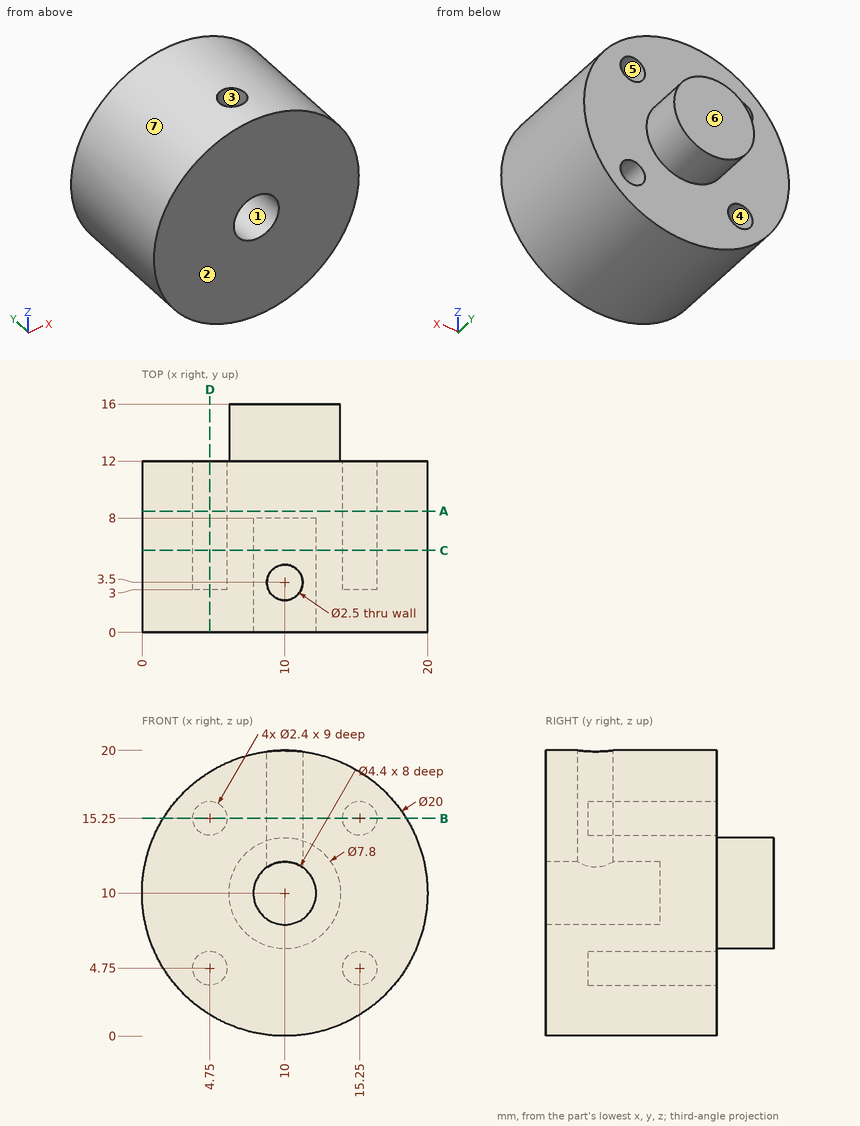
Study the drawing (mm; zero at the part's minimum x, y, z) and answer. A direction names the side the tool comes from. Give positions to 0.01 mm unless a question says otherwise; leave off trailing zeros. Write each loop counter-clockwise with the first axis right and the second up, starting at its lowest first coordinate (ties: lowest second). Pieces come first, ordered by that corner, then holes. Notation, with made-up numbers: (-11.75, 75) -> (19.25, 75) arc R30 ccw to (19.25, 106) -> close; hole circle Ø9 at (38, 75). An arc over 180 degrees is marked (long way). Write item = value, one per line. Start each with the question number.
1) Determine the mould class of the marked faces 5, 6 and 7 for opening direction X: +X half, -X half, draft (parallel to the pull), parting line (faces both ways), or undercut.
2) Each of these flat-tipped pins is pushed along its axis until it touches: pin 1 (5 mm diameter, centred on y = 7.5, z = 14, fed in from -X); pin 2 (1.9 mm diameter, centred on x = 4.75, z = 15.25, fed in from +Y); pin 3 (6 mm diameter, centred on x = 5.5, y = 7.5, fed in from -Z); pin 4 (5.5 mm diameter, centred on x = 10, z = 10, fed in from -Y). Where does it stop, or does it pass through?
3) The part is cut by section D-D, the plane x = 4.75. Determine the outline of the cut face in (y, z).
4) The part is cut by section A-A, the plane y = 8.5. Determine the outline of the cut face in (x, z), and give its area (3 significant figures).
5) The part is cut by section C-C, the plane y = 5.75. Determine the outline of the cut face in (x, z), and give its area (3 significant figures).
6) The part is cut by section B-B, the plane z = 15.25. Determine the outline of the cut face in (x, y), and give its area (3 significant figures).
7) Straight lines are drawn through the part: line 1 along Y through (x, z) = (10, 16.5); line 2 along Z through (x, y) = (4.75, 5.25); line 3 along Y through (x, z) = (8, 2). For each, find the intervals that lie inside material, in ascending order.
8) Which of the six approach directions +Z, -Z, +X, -X, +Y, -Y give full straight-line access (tool end or side, diameter ignored) to the marked faces 1, 2, 3 and 4?
Solutions:
q1.face_5 = undercut
q1.face_6 = draft
q1.face_7 = parting line
q2.pin_1 = 0.11
q2.pin_2 = 3
q2.pin_3 = 0.11
q2.pin_4 = 0
q3.outline = (0, 1.49) -> (12, 1.49) -> (12, 3.55) -> (3, 3.55) -> (3, 5.95) -> (12, 5.95) -> (12, 14.05) -> (3, 14.05) -> (3, 16.45) -> (12, 16.45) -> (12, 18.51) -> (0, 18.51) -> close
q4.outline = circle Ø20 at (10, 10); hole circle Ø2.4 at (4.75, 4.75); hole circle Ø2.4 at (4.75, 15.25); hole circle Ø2.4 at (15.25, 4.75); hole circle Ø2.4 at (15.25, 15.25)
q4.area = 296 mm²
q5.outline = circle Ø20 at (10, 10); hole circle Ø2.4 at (4.75, 4.75); hole circle Ø2.4 at (4.75, 15.25); hole circle Ø4.4 at (10, 10); hole circle Ø2.4 at (15.25, 4.75); hole circle Ø2.4 at (15.25, 15.25)
q5.area = 281 mm²
q6.outline = (1.49, 0) -> (18.51, 0) -> (18.51, 12) -> (16.45, 12) -> (16.45, 3) -> (14.05, 3) -> (14.05, 12) -> (5.95, 12) -> (5.95, 3) -> (3.55, 3) -> (3.55, 12) -> (1.49, 12) -> close; hole circle Ø2.5 at (10, 3.5)
q6.area = 156 mm²
q7.line_1 = 0 to 2.25, 4.75 to 12
q7.line_2 = 1.49 to 3.55, 5.95 to 14.05, 16.45 to 18.51
q7.line_3 = 0 to 12
q8.face_1 = -Y
q8.face_2 = +Z, -Z, +X, -X, -Y
q8.face_3 = +Z
q8.face_4 = +Y
